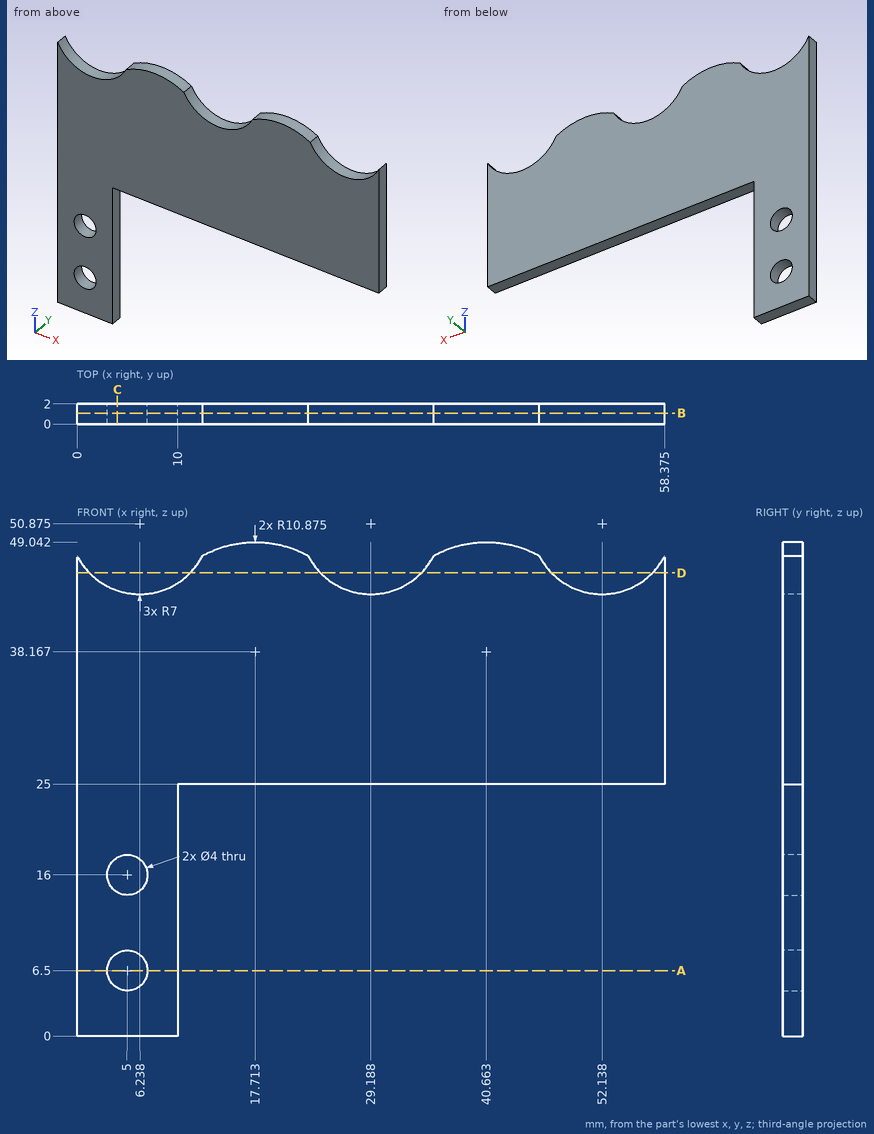
Here's the drawing with two shaded views (mm, measured from the low corner). I have some questions. Coordinates: 2 decimals unless noted, no trailing zeros. Loops run counter-clockwise (first coordinate to the right, second up) from the corner with the lowest first, then second, coordinate; pieces in that order, holes last. Notation, with made-up numbers: (-14, 15) -> (17, 15) arc R4 ccw to (17, 19) -> close; hole circle Ø9 at (89, 82). An arc over 180 degrees is marked (long way). Answer in a Markdown table with one row per item.
(1) If I drill on probe 1 along X at (y, z) = (1.8, 16); probe 2 along Z at (x, y) = (4, 1.7); probe 3 along Z at (x, y) = (52, 0.7), over which ranges is the centre line in solid material (lowest first)?
Results found:
| item | result |
|---|---|
| probe 1 | x = 0 to 3, 7 to 10 |
| probe 2 | z = 0 to 4.77, 8.23 to 14.27, 17.73 to 44.24 |
| probe 3 | z = 25 to 43.88 |
(2) Will these pins go through, and if not, where does the flat tip stop? pin 1 Ø0.6 at (x, y) = (36.5, 1) entering from -Z; pin 2 Ø5 at (x, z) = (5, 16) entering from +Y.
Results found:
| item | result |
|---|---|
| pin 1 | stops at z = 25 |
| pin 2 | stops at y = 2 |
(3) Imagine slicing it at D-D (z = 46). List the corners of the cut face in (x, y) for me (1 decimal).
Results found:
| item | result |
|---|---|
| outline | (0, 0) -> (1.2, 0) -> (1.2, 2) -> (0, 2) -> close; (11.3, 0) -> (24.2, 0) -> (24.2, 2) -> (11.3, 2) -> close; (34.2, 0) -> (47.1, 0) -> (47.1, 2) -> (34.2, 2) -> close; (57.2, 0) -> (58.4, 0) -> (58.4, 2) -> (57.2, 2) -> close |
(4) Imagine slicing it at B-B (y = 1.1). Give the number of separate pieces and of enclosed holes in the cut face, plus the area to 3 significant figures.
Results found:
| item | result |
|---|---|
| separate pieces | 1 |
| enclosed holes | 2 |
| area | 1,470 mm^2 |
(5) Imagine slicing it at C-C (x = 4). List the corners of the cut face in (y, z) for me.
Results found:
| item | result |
|---|---|
| outline | (0, 0) -> (2, 0) -> (2, 4.77) -> (0, 4.77) -> close; (0, 8.23) -> (2, 8.23) -> (2, 14.27) -> (0, 14.27) -> close; (0, 17.73) -> (2, 17.73) -> (2, 44.24) -> (0, 44.24) -> close |
(6) Imagine slicing it at A-A (z = 6.5). List the corners of the cut face in (x, y) for me.
Results found:
| item | result |
|---|---|
| outline | (0, 0) -> (3, 0) -> (3, 2) -> (0, 2) -> close; (7, 0) -> (10, 0) -> (10, 2) -> (7, 2) -> close |
